The figure shows three views and two pictorial views of one solid part (mm, origin at its lowest corner). Answer the questions. A direction names the side the tool comes from. Give positions to 0.01 mm unless a question says otherwise; leave off trailing zeros. Loops run counter-clockwise (first coordinate to the right, second up) from the corner with the lowest first, then second, coordinate; pieces in that order, holes last. Notation, with made-up numbers: M 42,-30.75 L 91,-30.75 A8 ccw 91,-25.75 Z; hole C -35,14.25 d1. An arc over 180 degrees is marked long. Answer as a JSON object with one key per item and string values. Group by question number.
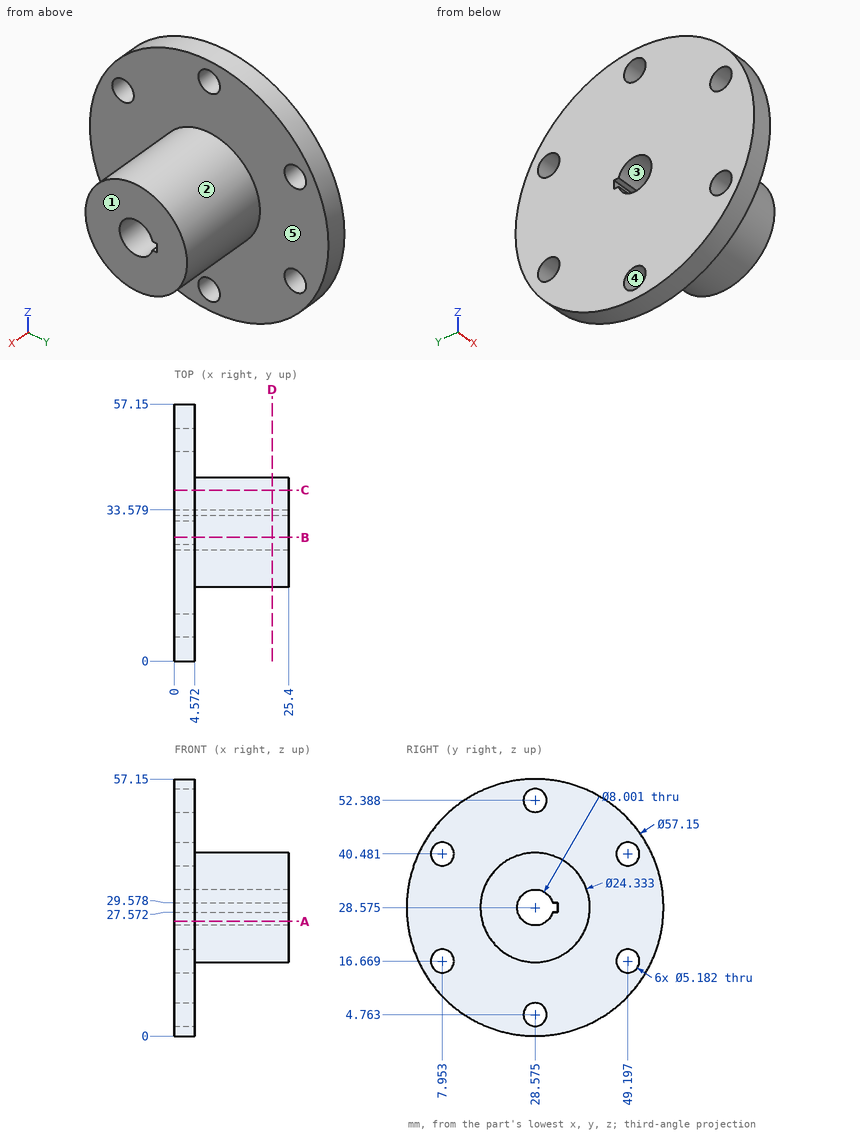
Item 1: A cutting plane is placed at A-A (z = 25.5). Determine the outline of the cut face in (x, y) (1 decimal), and give its area (3 significant figures).
Item 2: A cutting plane is placed at C-C (y = 38). Determine the outline of the cut face in (x, z).
Item 3: Given pin 1 Ø0.6 at (x, y) = (18.5, 33) entering from -Z; pin 2 Ø6 at (y, z) = (7.95, 40.48) entering from +X; pin 3 Ø5 at (x, z) = (3.5, 39.5) entering from -Y; pin 4 Ø4 at (y, z) = (28.58, 4.76) entering from -X, each flat-ended and moving along its own axis, determine where each tip first touches the part or whether it passes through.
Item 4: A tool of negligible diameter and unlimited length cuts with its end or side. For the marked faces 4 and 5, from which of +Z, -Z, +X, -X, +Y, -Y can it reach the whole face along a straight path? Write none if from no direction.
Item 5: Find the intervals of material crossed by probe 1 along X at (y, z) = (49.5, 45); probe 2 along Y at (x, z) = (2, 25.5) (1 decimal); probe 3 along Y at (x, z) = (2.5, 22.5), in increasing order. Write a range as [from, to].
Item 6: For a pull along Z with two mould halves and no side action, classify the marked faces 1, 2 and 3 as pulls with the +Z half, pulls with the -Z half, needs draft (parallel to the pull), parting line crosses it, or undercut.
Item 7: A cutting plane is placed at D-D (x = 21.75). Determine the outline of the cut face in (y, z) (1 decimal).
Item 8: A cutting plane is placed at B-B (y = 27.5). Determine the outline of the cut face in (x, z) (1 decimal).
The answers:
{
 "1": {"outline": "M 0,0.2 L 4.6,0.2 L 4.6,16.8 L 25.4,16.8 L 25.4,26 L 0,26 Z; M 0,31.1 L 25.4,31.1 L 25.4,40.3 L 4.6,40.3 L 4.6,57 L 0,57 Z", "area": "620 mm^2"},
 "2": {"outline": "M 0,1.6 L 4.57,1.6 L 4.57,20.88 L 25.4,20.88 L 25.4,36.27 L 4.57,36.27 L 4.57,55.55 L 0,55.55 Z"},
 "3": {"pin 1": "stops at z = 17.13", "pin 2": "stops at x = 4.57", "pin 3": "stops at y = 1.27", "pin 4": "passes through"},
 "4": {"face 4": "+X, -X", "face 5": "+X"},
 "5": {"probe 1": "x = [0, 4.57]", "probe 2": "y = [0.2, 26], [31.1, 57]", "probe 3": "y = [0.65, 56.5]"},
 "6": {"face 1": "needs draft", "face 2": "parting line crosses it", "face 3": "undercut"},
 "7": {"outline": "C 28.6,28.6 d24.3; hole M 32.4,27.6 L 33.6,27.6 L 33.6,29.6 L 32.4,29.6 A4 ccw long Z"},
 "8": {"outline": "M 0,0 L 4.6,0 L 4.6,2.4 L 0,2.4 Z; M 0,7.1 L 4.6,7.1 L 4.6,16.5 L 25.4,16.5 L 25.4,24.7 L 0,24.7 Z; M 0,32.4 L 25.4,32.4 L 25.4,40.7 L 4.6,40.7 L 4.6,50 L 0,50 Z; M 0,54.7 L 4.6,54.7 L 4.6,57.1 L 0,57.1 Z"}
}
